Work out the finished part from the listing and answer in its coordinate system (mm). Round coordinates to 2 decimals unless told otherwise and drop trailing zeros. Order: outer loops, then holes, each group sorted by start corner. A loop starts at its lowest first (then second) coordinate and runs counter-clockwise, first axis right, second up. Notation, with made-up numbers: (77.25, 64) - (103.25, 64) arc R21 ccw to (103.25, 100) - close; hole circle Ø2 at (55.5, -36.5). An arc over 180 degrees is marked (long way). Use one line per item in the form item = value. Start each with the question number.
Q1. Given P1, Ø1.5, axis at x = 3, y = 2, coming from the +Z side; P2, Ø1.5, axis at y = 1.5, z = -3.5, coming from the +X side, each flat-ended and moving along its own axis, determine where each tip first touches the part or whether it passes through.
Q2. Find the intervals of material crossed by line 1 (X direction, y = 2.85, z = -34); line 2 (Z direction, x = 62, y = 0.9) (3 decimals); line 3 (X direction, y = 1.55, z = -20), in increasing order. Write a range as [from, to].
Q3. The part is cut by section A-A on y = 1.3. Determine the outline of the cut face in (x, z).
from build123d import *

# Parameters (mm, degrees)
SKETCH1_W           = 72
SKETCH1_H           = 42.7549792
BOSS_EXTRUDE1_DEPTH = 3
SKETCH2_R           = 1.8
CUT_EXTRUDE1_DEPTH  = 3
SKETCH3_W           = 10.743475017
SKETCH3_H           = 9.971995481
SKETCH3_W_2         = 11.428139851
SKETCH3_H_2         = 7.796989135
SKETCH3_H_3         = 2.175006346
CUT_EXTRUDE2_DEPTH  = 53


with BuildPart() as part:
    # Sketch1 → Boss-Extrude1 (new body)
    with BuildSketch(Plane(origin=(0, 0, 0), x_dir=(1, 0, 0), z_dir=(0, 1, 0))):
        with Locations((36, 21.3774896)):
            Rectangle(SKETCH1_W, SKETCH1_H)
    extrude(amount=BOSS_EXTRUDE1_DEPTH)

    # Sketch2 → Cut-Extrude1 (cut)
    with BuildSketch(Plane(origin=(0, 3, 0), x_dir=(1, 0, 0), z_dir=(0, 1, 0))):
        with Locations(Location((7.244076977, 20.809705714, 0), (0, 0, 270))):
            Circle(SKETCH2_R)
        with Locations(Location((63.234445615, 20.809705714, 0), (0, 0, 270))):
            Circle(SKETCH2_R)
        with Locations(Location((63.234445615, 33.7549792, 0), (0, 0, 270))):
            Circle(SKETCH2_R)
    extrude(amount=-CUT_EXTRUDE1_DEPTH, mode=Mode.SUBTRACT)

    # Sketch3 → Cut-Extrude2 (cut)
    with BuildSketch(Plane(origin=(0, 3, 0), x_dir=(1, 0, 0), z_dir=(0, 1, 0))):
        with Locations((5.371737509, 4.985997741)):
            Rectangle(SKETCH3_W, SKETCH3_H)
        with Locations((66.285930075, 6.073500914)):
            Rectangle(SKETCH3_W_2, SKETCH3_H_2)
        with Locations((66.285930075, 1.087503173)):
            Rectangle(SKETCH3_W_2, SKETCH3_H_3)
    extrude(amount=-CUT_EXTRUDE2_DEPTH, mode=Mode.SUBTRACT)


solid = part.part
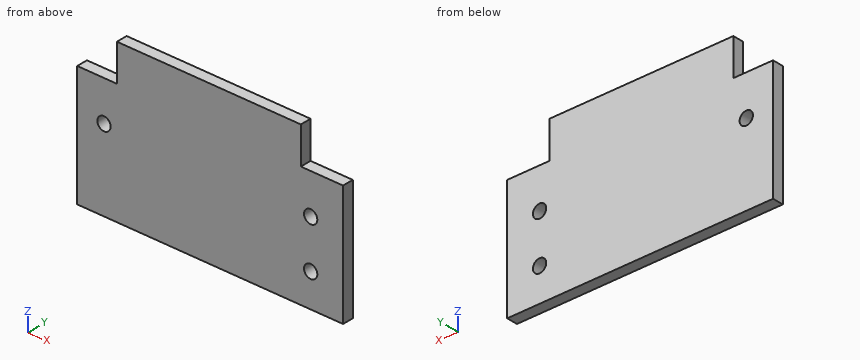
Found:
q1.P1 = -9.97
q1.P2 = 60.57
q2.line_1 = [0, 61.45], [65.02, 72]
q2.line_2 = [-42.755, -35.065], [-32.445, -22.12], [-19.5, -9.972]
q2.line_3 = [0, 5.64], [8.85, 61.63], [64.84, 72]
q3.outline = (0, -42.75) - (72, -42.75) - (72, -9.97) - (60.57, -9.97) - (60.57, 0) - (10.74, 0) - (10.74, -9.97) - (0, -9.97) - close; hole circle Ø3.6 at (7.24, -20.81); hole circle Ø3.6 at (63.23, -33.75); hole circle Ø3.6 at (63.23, -20.81)
